Read the model definition and answer for the solid it produces. Units are mm, in the model's axes. Face numbers are marked on the shaded views. A direction names the side the tool comes from. Coordinates: 2 decimals unless noted, no trailing zeros. Loops run counter-clockwise (first coordinate to the right, second up) from the corner with the lowest first, then second, coordinate; pieces in that order, holes last.
from build123d import *

# Parameters (mm, degrees)
SKETCH1_W           = 160
SKETCH1_H           = 95
BOSS_EXTRUDE1_DEPTH = 4.5
SKETCH2_R           = 1.5
CUT_EXTRUDE1_DEPTH  = 5
SKETCH5_W           = 160
SKETCH5_H           = 4.5
BOSS_EXTRUDE2_DEPTH = 135.5
SKETCH7_R           = 1.25
CUT_EXTRUDE2_DEPTH  = 5
SKETCH9_R           = 10.5
SKETCH9_R_2         = 5
SKETCH9_R_3         = 1.4
CUT_EXTRUDE3_DEPTH  = 5
SKETCH10_R          = 2.375
CUT_EXTRUDE4_DEPTH  = 10


with BuildPart() as part:
    # Sketch1 → Boss-Extrude1 (new body)
    with BuildSketch(Plane(origin=(0, 0, 0), x_dir=(1, 0, 0), z_dir=(0, 1, 0))):
        Rectangle(SKETCH1_W, SKETCH1_H)
    extrude(amount=BOSS_EXTRUDE1_DEPTH)

    # Sketch2 → Cut-Extrude1 (cut)
    with BuildSketch(Plane(origin=(0, 4.5, 0), x_dir=(1, 0, 0), z_dir=(0, 1, 0))):
        with Locations(Location((76, -21.5, 0), (0, 0, 270))):
            Circle(SKETCH2_R)
        with Locations(Location((-76, -21.5, 0), (0, 0, 270))):
            Circle(SKETCH2_R)
        with Locations(Location((-76, 43.5, 0), (0, 0, 270))):
            Circle(SKETCH2_R)
        with Locations(Location((76, 43.5, 0), (0, 0, 270))):
            Circle(SKETCH2_R)
    extrude(amount=-CUT_EXTRUDE1_DEPTH, mode=Mode.SUBTRACT)

    # Sketch5 → Boss-Extrude2 (add)
    with BuildSketch(Plane(origin=(0, 4.5, 0), x_dir=(1, 0, 0), z_dir=(0, 1, 0))):
        with Locations((0, -45.25)):
            Rectangle(SKETCH5_W, SKETCH5_H)
    extrude(amount=BOSS_EXTRUDE2_DEPTH)

    # Sketch7 → Cut-Extrude2 (cut)
    with BuildSketch(Plane(origin=(0, 0, 43), x_dir=(-1, 0, 0), z_dir=(0, 0, -1))):
        with Locations((76, 136)):
            Circle(SKETCH7_R)
        with Locations((-76, 136)):
            Circle(SKETCH7_R)
        with Locations((-76, 56)):
            Circle(SKETCH7_R)
        with Locations((76, 56)):
            Circle(SKETCH7_R)
    extrude(amount=-CUT_EXTRUDE2_DEPTH, mode=Mode.SUBTRACT)

    # Sketch9 → Cut-Extrude3 (cut)
    with BuildSketch(Plane(origin=(0, 4.5, 0), x_dir=(1, 0, 0), z_dir=(0, 1, 0))):
        with Locations((0, 42)):
            Circle(SKETCH9_R)
        with Locations(Location((-45.917706268, 40.60591365, 0), (0, 0, 270))):
            Circle(SKETCH9_R_2)
        with Locations(Location((-28.55, 43.75, 0), (0, 0, 270))):
            Circle(SKETCH9_R_3)
        with Locations(Location((-55.25, 30.17, 0), (0, 0, 270))):
            Circle(SKETCH9_R_3)
    extrude(amount=-CUT_EXTRUDE3_DEPTH, mode=Mode.SUBTRACT)

    # Sketch10 → Cut-Extrude4 (cut)
    with BuildSketch(Plane(origin=(0, 0, 43), x_dir=(-1, 0, 0), z_dir=(0, 0, -1))):
        with Locations((0, 8.4)):
            Circle(SKETCH10_R)
        with Locations((0, 38.4)):
            Circle(SKETCH10_R)
        with Locations((0, 67.6)):
            Circle(SKETCH10_R)
        with Locations((0, 127.6)):
            Circle(SKETCH10_R)
        with Locations((-50, 24)):
            Circle(SKETCH10_R)
        with Locations((50, 24)):
            Circle(SKETCH10_R)
    extrude(amount=-CUT_EXTRUDE4_DEPTH, mode=Mode.SUBTRACT)


solid = part.part
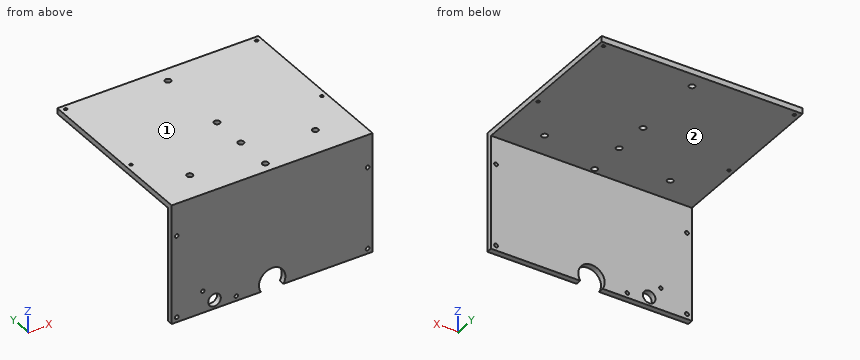
Q1. A cutting plane is placed at D-D (x = -20). Give the vertices of the cut face in (y, z).
Findings below:
outline: (0, -47.5) - (4.5, -47.5) - (4.5, 43) - (140, 43) - (140, 47.5) - (0, 47.5) - close
Q2. A cutting plane is placed at C-C (y = 24). Give the vertices of the cut face in (x, z) (3 decimals), then the cut area to 3 significant figures.
Findings below:
outline: (-80, 43) - (-52.375, 43) - (-52.375, 47.5) - (-80, 47.5) - close; (-47.625, 43) - (47.625, 43) - (47.625, 47.5) - (-47.625, 47.5) - close; (52.375, 43) - (80, 43) - (80, 47.5) - (52.375, 47.5) - close
area: 677 mm2
Q3. A cutting plane is placed at B-B (y = 38.4). Give the vertices of the cut face in (x, z) (3 decimals).
Findings below:
outline: (-80, 43) - (-2.375, 43) - (-2.375, 47.5) - (-80, 47.5) - close; (2.375, 43) - (80, 43) - (80, 47.5) - (2.375, 47.5) - close
Q4. Straight lines are drawn through the part: probe 1 along Z at (x, y) = (76, 3.4); probe 2 along Y at (x, z) = (0, 46) (3 decimals); probe 3 along Z at (x, y) = (0, 45). For each, find the intervals that lie inside material, in ascending order.
Findings below:
probe 1: z = -47.5 to -45, -42 to 20, 23 to 47.5
probe 2: y = 0 to 6.025, 10.775 to 36.025, 40.775 to 65.225, 69.975 to 125.225, 129.975 to 140
probe 3: z = 43 to 47.5
Q5. Flat-ended cylindrical pins translate along their axes: pin 1 Ø6 at (x, z) = (-28.5, -37.5) entering from -Y; pin 2 Ø11.5 at (x, z) = (-45.92, -40.61) entering from +Y; pin 3 Ø4.5 at (x, y) = (0, 38.4) entering from -Z (3 decimals); pin 4 Ø2 at (x, y) = (57.5, 37) entering from -Z. Find the tip coordinate at first contact, or state that the pin passes through.
Findings below:
pin 1: stops at y = 0
pin 2: stops at y = 4.5
pin 3: passes through
pin 4: stops at z = 43
Q6. Which of the six approach directions +Z, -Z, +X, -X, +Y, -Y give full straight-line access (tool end or side, diameter ignored) to the marked faces 1 and 2?
Findings below:
face 1: +Z, +X, -X, +Y, -Y
face 2: -Z, +X, -X, +Y
Q7. A cutting plane is placed at A-A (x = 0). Give the vertices of the cut face in (y, z) (3 decimals).
Findings below:
outline: (0, -31.5) - (4.5, -31.5) - (4.5, 43) - (6.025, 43) - (6.025, 47.5) - (0, 47.5) - close; (10.775, 43) - (36.025, 43) - (36.025, 47.5) - (10.775, 47.5) - close; (40.775, 43) - (65.225, 43) - (65.225, 47.5) - (40.775, 47.5) - close; (69.975, 43) - (125.225, 43) - (125.225, 47.5) - (69.975, 47.5) - close; (129.975, 43) - (140, 43) - (140, 47.5) - (129.975, 47.5) - close
